Geometry: final body of the model. Coordinates: model frame, mm. Give positions to 0.01 mm unless a question says otherwise; leave off trailing zeros. Write each loop counter-clockwise with the first axis right and the second up, starting at its lowest first coordinate (ties: lowest second). Pieces come first, ordered by that corner, then holes.
from build123d import *

# Parameters (mm, degrees)
F2_T     = -3.5
F3_R     = 1.74999
F4_R     = 38.25
F5_DEPTH = 3
F6_R     = 1.74999


# Not quite as in the source:
# - a fillet or chamfer that OpenCascade refuses, or shapes differently, is made with other operations: its cross-section is extruded or revolved along the edge and cut away or added
# - a fillet or chamfer is up to 0.001 mm smaller than in the source, because OpenCascade refuses the exact size


with BuildPart() as f1:
    # F0 (on Front) → F1 (revolve)
    with BuildSketch(Plane.XZ):
        with BuildLine():
            Line((0, 100), (0, 0))
            Line((0, 0), (40, 0))
            Line((40, 0), (40, 9.3798986314))
            add(Edge.make_bspline(
                [(40, 9.3798986314), (36.3615811377, 9.5180089921), (32.7559413641, 9.8779920191), (29.1503015906, 10.237975046)],
                knots=[0.9214250826, 0.9214250826, 0.9214250826, 0.9214250826, 1, 1, 1, 1], degree=3))
            Line((29.1503015906, 10.237975046), (30.0444061749, 19.1934501913))
            add(Edge.make_bspline(
                [(40, 18.3365735612), (39.0117054739, 18.370443261), (36.643767227, 18.4954262507), (33.3320197728, 18.8677992603), (31.0010337577, 19.1072868184), (30.0444061749, 19.1934501913)],
                knots=[113.3617815831, 113.3617815831, 113.3617815831, 113.3617815831, 116.3275721529, 120.4741421163, 123.3563956747, 123.3563956747, 123.3563956747, 123.3563956747], degree=3))
            Line((40, 18.3365735612), (40, 73.0902536278))
            add(Edge.make_bspline(
                [(31.7338511682, 71.8869126854), (32.4007501321, 71.9844232047), (34.386427689, 72.278853309), (37.1398587874, 72.6929898238), (39.229939508, 72.9860445189), (40, 73.0902536278)],
                knots=[0, 0, 0, 0, 2.0219920564, 6.0221045926, 8.3532693238, 8.3532693238, 8.3532693238, 8.3532693238], degree=3))
            Line((31.7338511682, 71.8869126854), (30.4177049547, 80.7901546359))
            add(Edge.make_bspline(
                [(30.4177049547, 80.7901546359), (33.6321840052, 81.2653438371), (36.8466630556, 81.7405330383), (40, 82.1441317937)],
                knots=[0, 0, 0, 0, 0.0502198484, 0.0502198484, 0.0502198484, 0.0502198484], degree=3))
            Line((40, 82.1441317937), (40, 100))
            Line((40, 100), (0, 100))
        make_face()
        with BuildLine():
            Line((40, 73.0902536278), (40, 82.1441317937))
            add(Edge.make_bspline(
                [(30.4177049547, 80.7901546359), (33.6321840052, 81.2653438371), (36.8466630556, 81.7405330383), (40, 82.1441317937)],
                knots=[0, 0, 0, 0, 0.0502198484, 0.0502198484, 0.0502198484, 0.0502198484], degree=3))
            Line((30.4177049547, 80.7901546359), (31.7338511682, 71.8869126854))
            add(Edge.make_bspline(
                [(31.7338511682, 71.8869126854), (32.4007501321, 71.9844232047), (34.386427689, 72.278853309), (37.1398587874, 72.6929898238), (39.229939508, 72.9860445189), (40, 73.0902536278)],
                knots=[0, 0, 0, 0, 2.0219920564, 6.0221045926, 8.3532693238, 8.3532693238, 8.3532693238, 8.3532693238], degree=3))
        make_face()
        with BuildLine():
            add(Edge.make_bspline(
                [(40, 9.3798986314), (36.3615811377, 9.5180089921), (32.7559413641, 9.8779920191), (29.1503015906, 10.237975046)],
                knots=[0.9214250826, 0.9214250826, 0.9214250826, 0.9214250826, 1, 1, 1, 1], degree=3))
            Line((40, 9.3798986314), (40, 18.3365735612))
            add(Edge.make_bspline(
                [(40, 18.3365735612), (39.0117054739, 18.370443261), (36.643767227, 18.4954262507), (33.3320197728, 18.8677992603), (31.0010337577, 19.1072868184), (30.0444061749, 19.1934501913)],
                knots=[113.3617815831, 113.3617815831, 113.3617815831, 113.3617815831, 116.3275721529, 120.4741421163, 123.3563956747, 123.3563956747, 123.3563956747, 123.3563956747], degree=3))
            Line((30.0444061749, 19.1934501913), (29.1503015906, 10.237975046))
        make_face()
    revolve(axis=Axis((0, 0, 50), (0, 0, 1)))

    # F2
    f2_openings = [f1.faces().sort_by_distance(p)[0] for p in [
        (0, 0, 100),
    ]]
    offset(amount=F2_T, openings=f2_openings)

    # F3 (radius 1.75 in the source; OpenCascade refuses exactly that, so slightly less here)
    f3_edges = [f1.edges().sort_by_distance(p)[0] for p in [
        (-40, 0, 100),
        (-36.5, 0, 100),
    ]]
    fillet(f3_edges, radius=F3_R)

    # F4 (on Top) → F5 (cut)
    with BuildSketch(Plane.XY):
        Circle(F4_R)
    extrude(amount=F5_DEPTH, mode=Mode.SUBTRACT)

    # F6 (radius 1.75 in the source; OpenCascade refuses exactly that, so slightly less here)
    f6_edges = [f1.edges().sort_by_distance(p)[0] for p in [
        (-40, 0, 0),
    ]]
    fillet(f6_edges, radius=F6_R)

    # F7: fillet of radius 5 on 1 edges, made by hand

    # F7_s1 → F7_t2 (revolve)
    with BuildSketch(Plane.XZ):
        with BuildLine():
            ThreePointArc((38.25, 0), (36.4060370926, 2.1833001327), (33.667424305, 3))
            Line((33.667424305, 3), (38.25, 3))
            Line((38.25, 3), (38.25, 0))
        make_face()
    revolve(axis=Axis((0, 0, 3), (0, 0, 1)))


solid = f1.part
Q1. Ray query, line 1 along Y through (x, z) = (0, 56); line 2 along X through (y, z) = (-1, 74.5); line 3 along Z through (x, y) = (8.5, -12). Return the intervals inside material, ascending.
Filled sheet:
line 1: y = -40 to -36.5, 36.5 to 40
line 2: x = -39.99 to -36.49, 36.49 to 39.99
line 3: z = 3 to 3.5
Q2. Section B-B on z = 42. Output: boundary loops of the cut face in (x, y), plus the area to 3 significant figures.
Filled sheet:
outline: circle Ø80 at (0, 0); hole circle Ø73 at (0, 0)
area: 841 mm2
Q3. Pin query (flat end, axial travel): P1, Ø10, axis at x = -5.5, z = 31.5, coming from the +Y side; P2, Ø1.5, axis at x = -31.5, y = 24.5, coming from the +Z side; P3, Ø1, axis at y = -31.5, z = 35, coming from the -X side. Return the tip coordinate at first contact, or that it passes through.
Filled sheet:
P1: stops at y = 40
P2: stops at z = 99.75
P3: stops at x = -25.28
Q4. Pull-direction query (Y, two-part tool) for faces 1 (the cylindrical face through (-7.912, -35.632, 51.538)), 2 (the cylindrical face through (-8.67, -39.05, 50.68)), 3 (the flat face through (0, 0, 3)); classes: released by +Y, released by -Y, zero draft, split by the parting line, or undercut.
Filled sheet:
face 1: undercut
face 2: split by the parting line
face 3: undercut
